Model file for the job. Use its own axes, mm. Round coordinates to 2 decimals unless told otherwise and drop trailing zeros. Order: outer loops, then holes, each group sorted by start corner. A loop starts at its lowest first (then second) coordinate and runs counter-clockwise, first axis right, second up. Notation, with made-up numbers: (70.5, 73) - (113.5, 73) arc R7 cw to (113.5, 83) - close; hole circle Ø9 at (-35.5, 7.25). An arc over 180 degrees is marked (long way). Put each result on its own line as item: value. Start each with the question number.
Item 1: Pin check, flat tips, straight feed: pin 1 Ø1 at (y, z) = (5.5, 0.5) entering from -X; pin 2 Ø2 at (x, z) = (-2, 3.5) entering from -Y. Stop position of each tip, or through.
Item 2: Saw through at C-C on z = 3.85. List the corners of the cut face in (x, y), plus the area to 3 significant figures.
Item 3: Probe probe 1 along Y at (x, z) = (0, 1); probe 2 along X at (y, z) = (-7.5, 3.2); probe 3 along X at (y, z) = (4.25, 1.95). List the from-to ranges inside material, lowest first.
Item 4: Saw through at A-A on y = 0. List the corners of the cut face in (x, z).
Item 5: Mould opens along X. For faces 1 (the face through (9, -5, 0)), 2 (the face through (-2.17, -9.76, 2.22)), 3 (the face through (12.356, -7.534, 2.218)), 4 (the face through (15.255, -6.996, 2.218)) say: pulls with the +X half, pulls with the -X half, needs draft (parallel to the pull), parting line crosses it, or undercut.
```python
from build123d import *

# Parameters (mm, degrees)
ESQUISSE1_R        = 10
BOSS_EXTRU_3_DEPTH = 4.5


with BuildPart() as part:
    # Esquisse1 → Boss.-Extru.3 (new body)
    with BuildSketch(Plane.XY):
        with BuildLine():
            Line((15.485185595, -5.176669047), (12.134231543, -3.650742984))
            ThreePointArc((12.134231543, -3.650742984), (12.035609724, -3.552721892), (12.024721053, -3.414100701))
            ThreePointArc((12.024721053, -3.414100701), (-11.374079439, 5.184623122), (10.464430261, -6.837082661))
            ThreePointArc((10.464430261, -6.837082661), (10.577237298, -6.754079946), (10.716830338, -6.765422852))
            Line((10.716830338, -6.765422852), (14.040747626, -8.325354826))
            ThreePointArc((14.040747626, -8.325354826), (14.40745115, -8.348324263), (14.690843755, -8.114470246))
            ThreePointArc((14.690843755, -8.114470246), (15.262737454, -6.979567539), (15.747114807, -5.80464408))
            ThreePointArc((15.747114807, -5.80464408), (15.739440197, -5.439232144), (15.485185595, -5.176669047))
        make_face()
        Circle(ESQUISSE1_R, mode=Mode.SUBTRACT)
    extrude(amount=BOSS_EXTRU_3_DEPTH)


solid = part.part
```
Results found:
1. pin 1: stops at x = -11.46
1. pin 2: stops at y = -12.46
2. outline: (10.46, -6.84) arc R0.2 cw to (10.72, -6.77) - (14.04, -8.33) arc R0.5 ccw to (14.69, -8.11) arc R16.78 ccw to (15.75, -5.8) arc R0.5 ccw to (15.49, -5.18) - (12.13, -3.65) arc R0.2 cw to (12.02, -3.41) arc R12.5 ccw (long way) to start; hole circle Ø20 at (0, 0)
2. area: 191 mm²
3. probe 1: y = -12.5 to -10, 10 to 12.5
3. probe 2: x = -10 to -6.61, 6.61 to 10, 12.28 to 15.01
3. probe 3: x = -11.76 to -9.05, 9.05 to 11.76
4. outline: (-12.5, 0) - (-10, 0) - (-10, 4.5) - (-12.5, 4.5) - close; (10, 0) - (12.5, 0) - (12.5, 4.5) - (10, 4.5) - close
5. face 1: needs draft
5. face 2: undercut
5. face 3: undercut
5. face 4: pulls with the +X half
